Verification items for the finished model (mm, model axes). Round coordinates to 2 decimals unless told otherwise and drop trailing zeros. Order: outer loops, then holes, each group sorted by start corner. A loop starts at its lowest first (then second) coordinate and runs counter-clockwise, first axis right, second up. Notation, with made-up numbers: M -3.5,15 L 42.5,15 A31 cw 42.5,48 Z; hole C 70,-14 d5. An arc over 180 degrees is marked long. Use CSV: the item, a comma, the result in double quotes. Start each with the question number.
Q1. Gauge pin test, flat ends, axial feed: pin 1 Ø0.6 at (x, y) = (-21.5, 0) entering from -Z; pin 2 Ø0.6 at (y, z) = (0, -0.5) entering from -X. Record the tip position at first contact, or that the pin passes through.
Q2. Sectioned sample at A-A (x = -16). Enter the section's corners in (y, z) (3 decimals).
Q3. Scan lines: line 1 (X direction, y = 0.25, z = -0.5); line 2 (Z direction, x = -10.25, y = -0.05); line 3 (Y direction, x = -21.5, z = -0.3). Record each from-to range of solid material in increasing order.
```python
from build123d import *

# Parameters (mm, degrees)
F2_R     = 0.994753
F3_DEPTH = 5.501


with BuildPart() as f1:
    # F0 (on Front) → F1 (revolve)
    with BuildSketch(Plane.XZ):
        Polygon((-25.386839, 0), (0, 0), (0, 0.625), (-16.636839, 0.625), (-16.636839, 0.375), (-18.136839, 0.375), (-18.136839, 0.63), (-19.636839, 0.63), (-19.636839, 0.4), (-19.886839, 0.4), (-19.886839, 0.56), (-22.976839, 0.56), (-23.286839, 0.25), (-25.136839, 0.25), align=None)
    revolve(axis=Axis((-12.69342, 0, 0), (-1, 0, 0)))

    # F2 (on face) → F3 (cut, through all)
    with BuildSketch(Plane.YZ.offset(-19.886839)):
        Circle(F2_R)
        Polygon((-0.41, 0.41), (0, 0.41), (0.41, 0.41), (0.41, 0), (0.41, -0.41), (0, -0.41), (-0.41, -0.41), (-0.41, 0), align=None, mode=Mode.SUBTRACT)
    extrude(amount=-F3_DEPTH, mode=Mode.SUBTRACT)


solid = f1.part
```
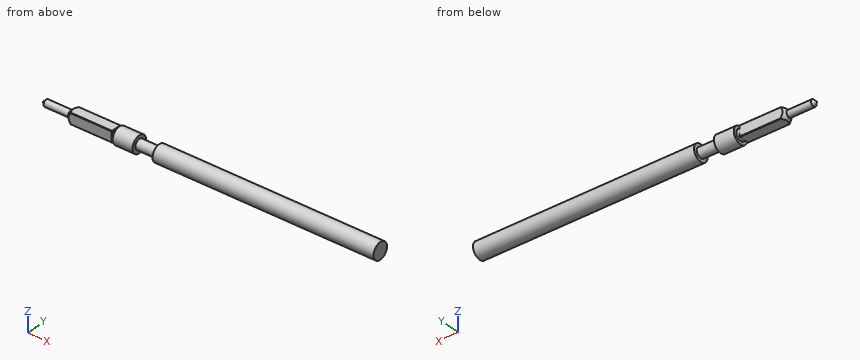
Verdict:
1,pin 1,"stops at z = -0.41"
1,pin 2,"stops at x = -25.19"
2,outline,"C 0,0 d1.25"
3,line 1,"x = -19.64 to -18.14, -16.64 to 0"
3,line 2,"z = -0.62 to 0.62"
3,line 3,"y = -0.41 to 0.41"
